The model under review builds one solid part; all positions refer to its coordinate system, in mm. Face numbers are marked on the shaded views. A direction names the side the tool comes from. Round coordinates to 2 decimals unless told otherwise and drop trailing zeros. Loops run counter-clockwise (first coordinate to the right, second up) from the corner with the lowest first, then second, coordinate; pieces in that order, holes last. Notation, with made-up numbers: M 60.5,61 L 109.5,61 A11 cw 109.5,79 Z; hole C 49.25,68 d7. An arc over 180 degrees is marked long. Return JSON: item names as keys, results as strings. Group by question number.
Q1. Consider section D-D (x = -1.5). State the section outline as (y, z) points.
Q2. For the marked faces 1, 2, 3, 4 and 5, list the 3-axis set-ups (+Z, -Z, +X, -X, +Y, -Y) from which the entire face can be reached by the end or side of a thin tool; tool diameter is ignored.
Q3. Consider section C-C (x = -11.75). State the section outline as (y, z) points, and give its area (3 significant figures).
Q4. To check wall thickness, follow line 1 along X through (y, z) = (10.25, 1.75); line 2 along Y through (x, z) = (-15.5, -2); line 3 along Z through (x, y) = (-8.75, -1). State the ranges of each line that lie inside material, in increasing order.
Q5. Clearance check with flat-ended pins moving along their axes: pin 1 Ø4.5 at (x, z) = (-14, -3.5) entering from -Y; pin 2 Ø1.5 at (x, y) = (-12.5, -0.5) entering from -Z; pin 3 Ø1.2 at (x, z) = (-10, -2.5) entering from +Y. State where each tip first meets the part, or that it passes through.
Q6. Consider section B-B (z = 0). State the section outline as (x, y) points.
Q7. Draft analysis for pull direction X (two halves, no side actions). For the marked faces 6, 7 and 8, state which applies: pulls with the +X half, pulls with the -X half, needs draft (parallel to the pull), parting line crosses it, or undercut.
Q8. Consider section A-A (y = 0). State the section outline as (x, z) points, and give its area (3 significant figures).
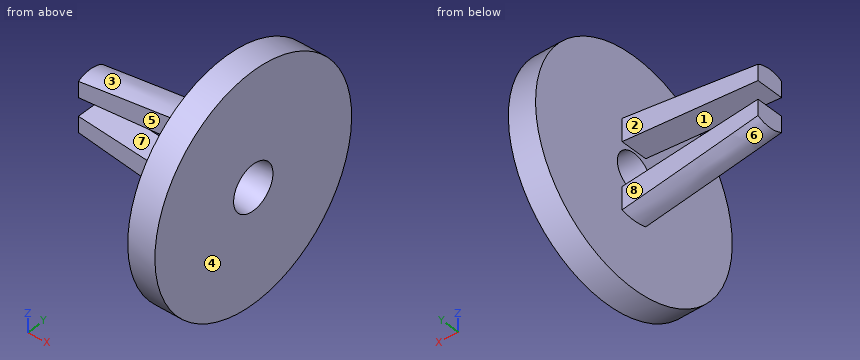
from build123d import *

# Parameters (mm, degrees)
F3_W     = 20
F3_H     = 4.5714285318
F4_DEPTH = 12.501
F5_DEPTH = 25
F7_DEPTH = 14.001


with BuildPart() as f2:
    # F0 (on Front) → F2 (revolve)
    with BuildSketch(Plane.XZ):
        Polygon((-18, 3.1265491901), (-18, 0.1), (0, 2.5), (0, 12.5), (-3, 12.5), (-3, 5.1265491901), align=None)
    revolve(axis=Axis((-8.8342446834, 0, 0), (-1, 0, 0)))

    # F3 (on Top) → F4 (cut, through all)
    with BuildSketch(Plane.XY):
        with Locations((-13, 3.7857142659)):
            Rectangle(F3_W, F3_H)
        with Locations((-13, -3.7857142659)):
            Rectangle(F3_W, F3_H)
    extrude(amount=F4_DEPTH, mode=Mode.SUBTRACT)

    # F3 (on Top) → F5 (cut)
    with BuildSketch(Plane.XY):
        with Locations((-13, 3.7857142659)):
            Rectangle(F3_W, F3_H)
        with Locations((-13, -3.7857142659)):
            Rectangle(F3_W, F3_H)
    extrude(amount=-F5_DEPTH, mode=Mode.SUBTRACT)

    # F6 (on face) → F7 (cut, through all)
    with BuildSketch(Plane.XZ.offset(1.5)):
        Polygon((-3, 0), (-3, 2.4047132604), (-18, 1), (-18, 0), (-18, -1), (-3, -2.4047132604), align=None)
    extrude(amount=-F7_DEPTH, mode=Mode.SUBTRACT)


solid = f2.part
Values:
{
 "1": {"outline": "C 0,0 d25; hole C 0,0 d4.6"},
 "2": {"face 1": "+Y, -Y", "face 2": "+Z, -Z, -X, +Y", "face 3": "+Z, -X", "face 4": "+Z, -Z, +X, +Y, -Y", "face 5": "+Z, -Z, -X, -Y"},
 "3": {"outline": "M -1.5,-3.66 A3.96 ccw 1.5,-3.66 L 1.5,-1.59 L -1.5,-1.59 Z; M -1.5,1.59 L 1.5,1.59 L 1.5,3.66 A3.96 ccw -1.5,3.66 Z", "area": "13.7 mm2"},
 "4": {"line 1": "x = -3 to 0", "line 2": "y = -1.5 to 1.5", "line 3": "z = -4.24 to -1.87, 1.87 to 4.24"},
 "5": {"pin 1": "stops at y = -1.5", "pin 2": "stops at z = -3.95", "pin 3": "stops at y = 1.5"},
 "6": {"outline": "M -3,-12.5 L 0,-12.5 L 0,-2.5 L -3,-2.1 Z; M -3,2.1 L 0,2.5 L 0,12.5 L -3,12.5 Z"},
 "7": {"face 6": "pulls with the -X half", "face 7": "undercut", "face 8": "needs draft"},
 "8": {"outline": "M -18,-3.13 L -3,-5.13 L -3,-12.5 L 0,-12.5 L 0,-2.5 L -3,-2.1 L -3,-2.4 L -18,-1 Z; M -18,1 L -3,2.4 L -3,2.1 L 0,2.5 L 0,12.5 L -3,12.5 L -3,5.13 L -18,3.13 Z", "area": "134 mm2"}
}
